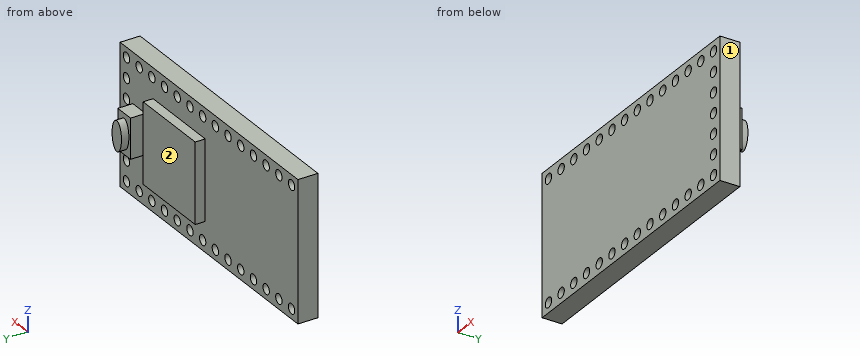
from build123d import *

# Parameters (mm, degrees)
SKETCH1_W           = 35.56
SKETCH1_H           = 17.78
BOSS_EXTRUDE1_DEPTH = 2.54
SKETCH2_R           = 0.635
CUT_EXTRUDE1_DEPTH  = 2.54
SKETCH3_W           = 2.54
SKETCH3_H           = 5.08
BOSS_EXTRUDE2_DEPTH = 1.905
SKETCH4_RX          = 1.905
SKETCH4_RY          = 0.9398
BOSS_EXTRUDE3_DEPTH = 0.9398
SKETCH5_W           = 10.414444886
SKETCH5_H           = 10.16
BOSS_EXTRUDE4_DEPTH = 1.27


with BuildPart() as part:
    # Sketch1 → Boss-Extrude1 (new body)
    with BuildSketch(Plane(origin=(0, 0, 0), x_dir=(1, 0, 0), z_dir=(0, 1, 0))):
        Rectangle(SKETCH1_W, SKETCH1_H)
    extrude(amount=BOSS_EXTRUDE1_DEPTH)

    # Sketch2 → Cut-Extrude1 (cut)
    with BuildSketch(Plane(origin=(0, 2.54, 0), x_dir=(1, 0, 0), z_dir=(0, 1, 0))):
        with Locations(Location((-16.51, 7.62, 0), (0, 0, 270))):
            Circle(SKETCH2_R)
        with Locations(Location((-16.51, -7.62, 0), (0, 0, 270))):
            Circle(SKETCH2_R)
        with Locations(Location((-13.97, 7.62, 0), (0, 0, 270))):
            Circle(SKETCH2_R)
        with Locations(Location((-13.97, -7.62, 0), (0, 0, 270))):
            Circle(SKETCH2_R)
        with Locations(Location((-11.43, 7.62, 0), (0, 0, 270))):
            Circle(SKETCH2_R)
        with Locations(Location((-11.43, -7.62, 0), (0, 0, 270))):
            Circle(SKETCH2_R)
        with Locations(Location((-8.89, 7.62, 0), (0, 0, 270))):
            Circle(SKETCH2_R)
        with Locations(Location((-8.89, -7.62, 0), (0, 0, 270))):
            Circle(SKETCH2_R)
        with Locations(Location((-6.35, 7.62, 0), (0, 0, 270))):
            Circle(SKETCH2_R)
        with Locations(Location((-6.35, -7.62, 0), (0, 0, 270))):
            Circle(SKETCH2_R)
        with Locations(Location((-3.81, 7.62, 0), (0, 0, 270))):
            Circle(SKETCH2_R)
        with Locations(Location((-3.81, -7.62, 0), (0, 0, 270))):
            Circle(SKETCH2_R)
        with Locations(Location((-1.27, 7.62, 0), (0, 0, 270))):
            Circle(SKETCH2_R)
        with Locations(Location((-1.27, -7.62, 0), (0, 0, 270))):
            Circle(SKETCH2_R)
        with Locations(Location((1.27, 7.62, 0), (0, 0, 270))):
            Circle(SKETCH2_R)
        with Locations(Location((1.27, -7.62, 0), (0, 0, 270))):
            Circle(SKETCH2_R)
        with Locations(Location((3.81, 7.62, 0), (0, 0, 270))):
            Circle(SKETCH2_R)
        with Locations(Location((3.81, -7.62, 0), (0, 0, 270))):
            Circle(SKETCH2_R)
        with Locations(Location((6.35, 7.62, 0), (0, 0, 270))):
            Circle(SKETCH2_R)
        with Locations(Location((6.35, -7.62, 0), (0, 0, 270))):
            Circle(SKETCH2_R)
        with Locations(Location((8.89, 7.62, 0), (0, 0, 270))):
            Circle(SKETCH2_R)
        with Locations(Location((8.89, -7.62, 0), (0, 0, 270))):
            Circle(SKETCH2_R)
        with Locations(Location((11.43, 7.62, 0), (0, 0, 270))):
            Circle(SKETCH2_R)
        with Locations(Location((11.43, -7.62, 0), (0, 0, 270))):
            Circle(SKETCH2_R)
        with Locations(Location((13.97, 7.62, 0), (0, 0, 270))):
            Circle(SKETCH2_R)
        with Locations(Location((13.97, -7.62, 0), (0, 0, 270))):
            Circle(SKETCH2_R)
        with Locations(Location((16.51, 7.62, 0), (0, 0, 270))):
            Circle(SKETCH2_R)
        with Locations(Location((16.51, -7.62, 0), (0, 0, 270))):
            Circle(SKETCH2_R)
        with Locations(Location((16.51, 5.08, 0), (0, 0, 270))):
            Circle(SKETCH2_R)
        with Locations(Location((16.51, 2.54, 0), (0, 0, 270))):
            Circle(SKETCH2_R)
        with Locations(Location((16.51, 0, 0), (0, 0, 270))):
            Circle(SKETCH2_R)
        with Locations(Location((16.51, -2.54, 0), (0, 0, 270))):
            Circle(SKETCH2_R)
        with Locations(Location((16.51, -5.08, 0), (0, 0, 270))):
            Circle(SKETCH2_R)
    extrude(amount=-CUT_EXTRUDE1_DEPTH, mode=Mode.SUBTRACT)

    # Sketch3 → Boss-Extrude2 (add)
    with BuildSketch(Plane(origin=(0, 2.54, 0), x_dir=(1, 0, 0), z_dir=(0, 1, 0))):
        with Locations((13.97, 0)):
            Rectangle(SKETCH3_W, SKETCH3_H)
    extrude(amount=BOSS_EXTRUDE2_DEPTH)

    # Sketch4 → Boss-Extrude3 (add)
    with BuildSketch(Plane(origin=(0, 4.445, 0), x_dir=(1, 0, 0), z_dir=(0, 1, 0))):
        with Locations(Location((13.97, 0), (0, 0, -90))):
            Ellipse(SKETCH4_RX, SKETCH4_RY)
    extrude(amount=BOSS_EXTRUDE3_DEPTH)

    # Sketch5 → Boss-Extrude4 (add)
    with BuildSketch(Plane(origin=(0, 2.54, 0), x_dir=(1, 0, 0), z_dir=(0, 1, 0))):
        with Locations((5.968777557, 0)):
            Rectangle(SKETCH5_W, SKETCH5_H)
    extrude(amount=BOSS_EXTRUDE4_DEPTH)


solid = part.part
Verification items for the finished model (mm, model axes). Face numbers are marked on the shaded views. A direction names the side the tool comes from. Coordinates: 2 decimals unless noted, no trailing zeros. Order: outer loops, then holes, each group sorted by start corner. A loop starts at its lowest first (then second) coordinate and runs counter-clockwise, first axis right, second up.
Item 1: Depth check by flat-ended pin: pin 1 (1.7 mm diameter, centred on x = 16.51, z = 5.08, fed in from +Y); pin 2 (1 mm diameter, centred on y = 3.5, z = 1, fed in from -X); pin 3 (1 mm diameter, centred on y = 3.5, z = -1, fed in from +X); pin 4 (1.1 mm diameter, centred on x = -6.35, z = 7.62, fed in from +Y). Enter the tip coordinate at first touch or a pass-through.
Filled in:
pin 1: stops at y = 2.54
pin 2: stops at x = 0.76
pin 3: stops at x = 15.24
pin 4: passes through
Item 2: Material ranges on L1, parallel to Z at x = -9, y = 1.75; L2, parallel to Y at x = 3.5, z = 8.25; L3, parallel to Y at x = 1, z = -4.75, recorded low to high.
Filled in:
L1: z = -8.89 to -8.25, -6.99 to 6.99, 8.25 to 8.89
L2: y = 0 to 2.54
L3: y = 0 to 3.81
Item 3: Section check C-C, the plane x = 1.27. Enter the section's corners in (y, z) (3 decimals).
Filled in:
outline: (0, -8.89) - (2.54, -8.89) - (2.54, -8.255) - (0, -8.255) - close; (0, -6.985) - (2.54, -6.985) - (2.54, -5.08) - (3.81, -5.08) - (3.81, 5.08) - (2.54, 5.08) - (2.54, 6.985) - (0, 6.985) - close; (0, 8.255) - (2.54, 8.255) - (2.54, 8.89) - (0, 8.89) - close
Item 4: Access from +Z, -Z, +X, -X, +Y, -Y to the whole of each face (thin tool, end or side, straight path). Record for the marked faces 1 and 2.
Filled in:
face 1: +Z, -Z, +X, +Y, -Y
face 2: +Z, -Z, -X, +Y
Item 5: Section check A-A, the plane x = -11.43. Enter the section's corners in (y, z) (3 decimals), then the cut area to 3 significant figures.
Filled in:
outline: (0, -8.89) - (2.54, -8.89) - (2.54, -8.255) - (0, -8.255) - close; (0, -6.985) - (2.54, -6.985) - (2.54, 6.985) - (0, 6.985) - close; (0, 8.255) - (2.54, 8.255) - (2.54, 8.89) - (0, 8.89) - close
area: 38.7 mm2
Item 6: Section check B-B, the plane y = 1.15. Give the number of separate pieces and of enclosed holes in the cut face, then the cut area to 3 significant figures.
Filled in:
separate pieces: 1
enclosed holes: 33
area: 590 mm2
